from build123d import *

# Parameters (mm, degrees)
BOSS_EXTRUDE1_DEPTH = 13
CUT_EXTRUDE1_DEPTH  = 26
BOSS_EXTRUDE3_DEPTH = 26
LPATTERN1_COUNT     = 5
LPATTERN1_PITCH     = 6
FILLET1_R           = 6
FILLET2_R           = 0.4
FILLET3_R           = 0.4
FILLET4_R           = 0.4
FILLET5_R           = 0.4
FILLET6_R           = 0.4
FILLET7_R           = 6
FILLET8_R           = 4
SKETCH4_R           = 1.5
CUT_EXTRUDE2_DEPTH  = 26
CUT_EXTRUDE3_DEPTH  = 7
SKETCH6_R           = 1.75
BOSS_EXTRUDE4_DEPTH = 1.5
SKETCH7_R           = 1.25
BOSS_EXTRUDE5_DEPTH = 0.5
CUT_EXTRUDE7_DEPTH  = 10


with BuildPart() as part:
    # Sketch1 → Boss-Extrude1 (new, symmetric)
    with BuildSketch(Plane(origin=(0, 0, 0), x_dir=(1, 0, 0), z_dir=(0, 1, 0))):
        Polygon((-26.537476469, 34.756624027), (-8.502257827, -32.880132907), (1.497742173, -32.349622066), (-2.834075277, 38.51810936), align=None)
        with BuildLine():
            Line((20.769613605, -36.051991051), (25.741983559, -27.375843459))
            ThreePointArc((25.741983559, -27.375843459), (23.519716976, -19.186732931), (15.330606448, -21.408999514))
            Line((15.330606448, -21.408999514), (10.358236494, -30.085147107))
            Line((10.358236494, -30.085147107), (1.497742173, -32.349622066))
            Line((1.497742173, -32.349622066), (-13.502257827, -33.145388327))
            Line((-13.502257827, -33.145388327), (-13.502257827, -43.145388327))
            Line((-13.502257827, -43.145388327), (-8.151905345, -54.993330272))
            Line((-8.151905345, -54.993330272), (9.769613605, -79.051991051))
            Line((9.769613605, -79.051991051), (9.769613605, -86.051991051))
            Line((9.769613605, -86.051991051), (20.769613605, -86.051991051))
            Line((20.769613605, -86.051991051), (20.769613605, -36.051991051))
        make_face()
    extrude(amount=BOSS_EXTRUDE1_DEPTH, both=True)

    # Sketch2 → Cut-Extrude1 (cut)
    with BuildSketch(Plane(origin=(0, 13, 0), x_dir=(1, 0, 0), z_dir=(0, 1, 0))):
        Polygon((0.878679347, -54.871314491), (15.878679347, -54.871314491), (15.878679347, -79.871314491), align=None)
    extrude(amount=-CUT_EXTRUDE1_DEPTH, mode=Mode.SUBTRACT)

    # Sketch3 → Boss-Extrude3 (add)
    with BuildSketch(Plane(origin=(0, 13, 0), x_dir=(1, 0, 0), z_dir=(0, 1, 0))):
        Polygon((20.769613605, -77.051991051), (20.769613605, -79.051991051), (24.769613605, -79.051991051), align=None)
        Polygon((20.769613605, -79.051991051), (20.769613605, -81.051991051), (24.769613605, -79.051991051), align=None)
    boss_extrude3 = extrude(amount=-BOSS_EXTRUDE3_DEPTH)

    # LPattern1: Boss-Extrude3 ×5
    with Locations(*[(0, 0, -i * LPATTERN1_PITCH) for i in range(1, LPATTERN1_COUNT)]):
        add(boss_extrude3)

    # Fillet1
    fillet1_edges = [part.edges().sort_by_distance(p)[0] for p in [
        (-26.537476469, 0, -34.756624027),
        (-2.834075277, 0, -38.51810936),
    ]]
    fillet(fillet1_edges, radius=FILLET1_R)

    # Fillet2
    fillet2_edges = [part.edges().sort_by_distance(p)[0] for p in [
        (24.769613605, 0, 79.051991051),
    ]]
    fillet(fillet2_edges, radius=FILLET2_R)

    # Fillet3
    fillet3_edges = [part.edges().sort_by_distance(p)[0] for p in [
        (24.769613605, 0, 73.051991051),
    ]]
    fillet(fillet3_edges, radius=FILLET3_R)

    # Fillet4
    fillet4_edges = [part.edges().sort_by_distance(p)[0] for p in [
        (24.769613605, 0, 67.051991051),
    ]]
    fillet(fillet4_edges, radius=FILLET4_R)

    # Fillet5
    fillet5_edges = [part.edges().sort_by_distance(p)[0] for p in [
        (24.769613605, 0, 61.051991051),
    ]]
    fillet(fillet5_edges, radius=FILLET5_R)

    # Fillet6
    fillet6_edges = [part.edges().sort_by_distance(p)[0] for p in [
        (24.769613605, 0, 55.051991051),
    ]]
    fillet(fillet6_edges, radius=FILLET6_R)

    # Fillet7
    # the kernel refuses this fillet: 6 mm, written as the material it takes off along each edge
    with BuildSketch(Plane(origin=(-13.502257827, -16.229856517, 43.145388327), x_dir=(0, 0, -1), z_dir=(0, 1, 0))) as fillet7_piece_1:
        with BuildLine():
            CenterArc((FILLET7_R * 0.215323767796, -FILLET7_R), FILLET7_R, 90, 24.303219814)
            Line((-FILLET7_R * 0.196241807704, -FILLET7_R * 0.0886198504117), (-FILLET7_R * 0.204473119214, -FILLET7_R * 0.0703922474199))
            Line((-FILLET7_R * 0.204473119214, -FILLET7_R * 0.0703922474199), (-FILLET7_R * 0.00430647535592, FILLET7_R * 0.02))
            Line((-FILLET7_R * 0.00430647535592, FILLET7_R * 0.02), (FILLET7_R * 0.215323767796, FILLET7_R * 0.02))
            Line((FILLET7_R * 0.215323767796, FILLET7_R * 0.02), (FILLET7_R * 0.215323767796, 0))
        make_face()
    extrude(amount=32.459713034, mode=Mode.SUBTRACT)
    with BuildSketch(Plane(origin=(-13.502257827, -27.127060907, 33.145388327), x_dir=(0.9985957546463174, 0, -0.052976587303748185), z_dir=(0, 1, 0))) as fillet7_piece_2_section:
        with BuildLine():
            CenterArc((5.692213138, -5.960748743), FILLET7_R, 96.557311778, 80.405931773)
            Line((-0.29936139, -5.642889219), (-0.419192881, -5.636532029))
            Line((-0.419192881, -5.636532029), (-0.119831491, 0.00635719))
            Line((-0.119831491, 0.00635719), (0, 0.12))
            ThreePointArc((0, 0.12), (2.50351555, 0.12), (4.993327459, 0.119214975))
            Line((4.993327459, 0.119214975), (5.0070311, 0))
        make_face()
    fillet7_piece_2 = extrude(amount=54.254121814, mode=Mode.PRIVATE)
    fillet7_piece_2 = split(fillet7_piece_2, bisect_by=Plane(origin=(-8.382183635, 0, 33.330442332), z_dir=(-0.9662393847687492, 0, 0.25764598060460653)), keep=Keep.TOP, mode=Mode.PRIVATE)
    add(fillet7_piece_2, mode=Mode.SUBTRACT)

    # Fillet8
    fillet8_edges = [part.edges().sort_by_distance(p)[0] for p in [
        (9.769613605, 0, 86.051991051),
    ]]
    fillet(fillet8_edges, radius=FILLET8_R)

    # Sketch4 → Cut-Extrude2 (cut)
    with BuildSketch(Plane(origin=(0, 13, 0), x_dir=(1, 0, 0), z_dir=(0, 1, 0))):
        with Locations(Location((-20.798923606, 30.81758039, 0), (0, 0, 270))):
            Circle(SKETCH4_R)
    extrude(amount=-CUT_EXTRUDE2_DEPTH, mode=Mode.SUBTRACT)

    # Sketch5 → Cut-Extrude3 (cut)
    with BuildSketch(Plane(origin=(-31.588699111, 0, 23.530714154), x_dir=(0.5973839650110779, 0, 0.8019553593234747), z_dir=(-0.8019553593234747, 0, 0.5973839650110779))):
        Polygon((67.232378401, 7.385302578), (46.232378401, 10.5), (46.232378401, -10), (67.232378401, -4.614697422), align=None)
    extrude(amount=-CUT_EXTRUDE3_DEPTH, mode=Mode.SUBTRACT)

    # Sketch6 → Boss-Extrude4 (add)
    with BuildSketch(Plane(origin=(0, 13, 0), x_dir=(1, 0, 0), z_dir=(0, 1, 0))):
        with Locations(Location((20.536295004, -24.392421487, 0), (0, 0, 270))):
            Circle(SKETCH6_R)
        with Locations(Location((-7.502257827, -43.116441091, 0), (0, 0, 270))):
            Circle(SKETCH6_R)
    boss_extrude4 = extrude(amount=BOSS_EXTRUDE4_DEPTH)

    # Sketch7 → Boss-Extrude5 (add)
    with BuildSketch(Plane(origin=(0, 14.5, 0), x_dir=(1, 0, 0), z_dir=(0, 1, 0))):
        with Locations(Location((-7.502257827, -43.116441091, 0), (0, 0, 270))):
            Circle(SKETCH7_R)
        with Locations(Location((20.536295004, -24.392421487, 0), (0, 0, 270))):
            Circle(SKETCH7_R)
    boss_extrude5 = extrude(amount=BOSS_EXTRUDE5_DEPTH)

    # Sketch8 → Cut-Extrude7 (cut)
    with BuildSketch(Plane(origin=(0, 15, 0), x_dir=(1, 0, 0), z_dir=(0, 1, 0))):
        with BuildLine():
            Line((-9.614117845, 23.451702753), (-1.459254761, -26.548297247))
            ThreePointArc((-1.459254761, -26.548297247), (-3.602858696, -29.527400736), (-6.581962185, -27.3837968))
            Line((-6.581962185, -27.3837968), (-14.736825269, 22.6162032))
            ThreePointArc((-14.736825269, 22.6162032), (-12.593221334, 25.595306688), (-9.614117845, 23.451702753))
        make_face()
    cut_extrude7 = extrude(amount=-CUT_EXTRUDE7_DEPTH, mode=Mode.SUBTRACT)

    # Mirror1: Boss-Extrude4, Boss-Extrude5, Cut-Extrude7 across plane
    add(boss_extrude4.mirror(Plane.ZX))
    add(boss_extrude5.mirror(Plane.ZX))
    add(cut_extrude7.mirror(Plane.ZX), mode=Mode.SUBTRACT)


solid = part.part
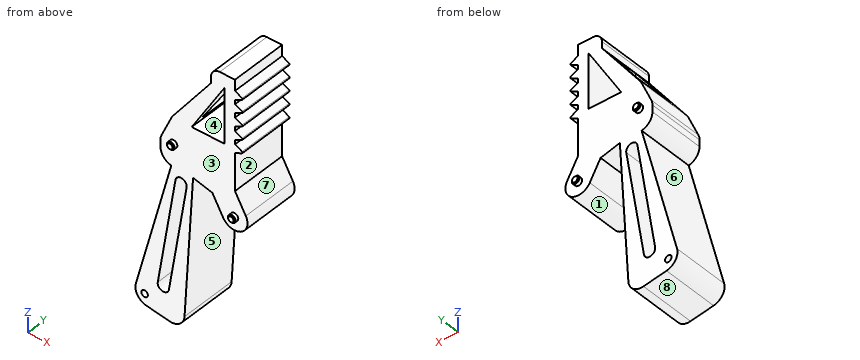
Input: part model. Units: mm. Frame: model coordinates. Face numbers are marked on the shaded views. A direction names the side the tool comes from. Round coordinates to 2 decimals unless told otherwise and drop trailing zeros. Order: outer loops, then holes, each group sorted by start corner. A loop starts at its lowest first (then second) coordinate and runs counter-clockwise, first axis right, second up. Notation, with made-up numbers: (71.25, 45.25) - (96.25, 45.25) arc R16 cw to (96.25, 66.25) - close; hole circle Ø8 at (68, 59.25). An arc over 180 degrees is marked (long way). Answer as a JSON object with one key per item and string values. Group by question number.
(1) Draft query along X for the marked faces 1, 2 and 3. Return one class per face: released by +X, released by -X, zero draft, split by the parting line, or undercut.
(2) Cut plane B-B (z = -7.5). Return loops of the section in (x, y).
(3) Cut plane C-C (x = 4). Return loops of the section in (y, z).
(4) Cut plane A-A (x = -11). Return loops of the section in (y, z).
(5) Pin query (flat end, axial travel): P1, Ø14.5, axis at x = -5, z = 12.5, coming from the -Y side; P2, Ø4, axis at x = -17, y = -9.5, coming from the -Z side; P3, Ø1.5, axis at x = -14.5, z = 6, coming from the +Y side. Return the tip coordinate at first contact, or that it passes through.
(6) Cut plane D-D (y = -6.5). Count the separate pieces of the cut face and the enclosed holes in it, then the cut area to 3 significant figures.
(7) Reachability of the marked faces 4, 5, 6, 7 and 8 from +Z, -Z, +X, -X, +Y, -Y: full face, straight path, thin tool, end or side. Return the list, or none.
(8) Material intervals for probe 1 along Y at (x, z) = (-5, -28.5); probe 2 along Z at (x, y) = (13.5, 0.5); probe 3 along Z at (x, y) = (21.5, -7), sorted ascending. Write a range as from..to.
Here are the results:
{
 "1": {"face 1": "undercut", "face 2": "released by +X", "face 3": "zero draft"},
 "2": {"outline": "(-19.27, -13) - (-12.27, -13) - (-12.27, -5) - (-7.01, -5) - (-7.01, -13) - (-0.94, -13) - (-0.94, 13) - (-7.01, 13) - (-7.01, 5) - (-12.27, 5) - (-12.27, 13) - (-19.27, 13) - close"},
 "3": {"outline": "(-13, 31.71) - (13, 31.71) - (13, 54.87) - (-13, 54.87) - close; (-13, 60.07) - (-8.89, 60.07) - (-6.58, 71.31) - (-13, 71.31) - close; (8.52, 71.31) - (9.86, 60.07) - (13, 60.07) - (13, 71.31) - close"},
 "4": {"outline": "(-13, -37.22) - (13, -37.22) - (13, -25.35) - (5, -25.35) - (5, 0.3) - (13, 0.3) - (13, 23.51) - (-13, 23.51) - (-13, 0.3) - (-5, 0.3) - (-5, -25.35) - (-13, -25.35) - close; (-13, 33.92) - (13, 33.92) - (13, 48.69) - (-13, 48.69) - close"},
 "5": {"P1": "stops at y = -13", "P2": "stops at z = -36.59", "P3": "stops at y = 13"},
 "6": {"separate pieces": "1", "enclosed holes": "2", "area": "2,110 mm^2"},
 "7": {"face 4": "+Y, -Y", "face 5": "-Z, +Y, -Y", "face 6": "-X, +Y, -Y", "face 7": "+X, +Y, -Y", "face 8": "-Z, -X, +Y, -Y"},
 "8": {"probe 1": "y = -13..13", "probe 2": "z = 24.6..54.87, 75.91..86.04", "probe 3": "z = 18.47..34.78, 53.42..56.69, 59.42..62.69, 65.42..68.69, 71.42..74.69, 77.42..80.69"}
}
